The drawing under review shows one solid part. Ordinate dimensions are in mm from its lowest x, y, z. Round coordinates to 2 decimals unless told otherwise and drop trailing zeros. Order: outer loops, then holes, each group sorted by start corner. A loop starts at its lowest first (then second) coordinate and runs counter-clockwise, first axis right, second up. Notation, with made-up numbers: M 76,74 L 108,74 A20 cw 108,105 Z; hole C 74.5,-4 d9. An arc over 180 degrees is marked long. Write item = value, one per line. Start each with the question number.
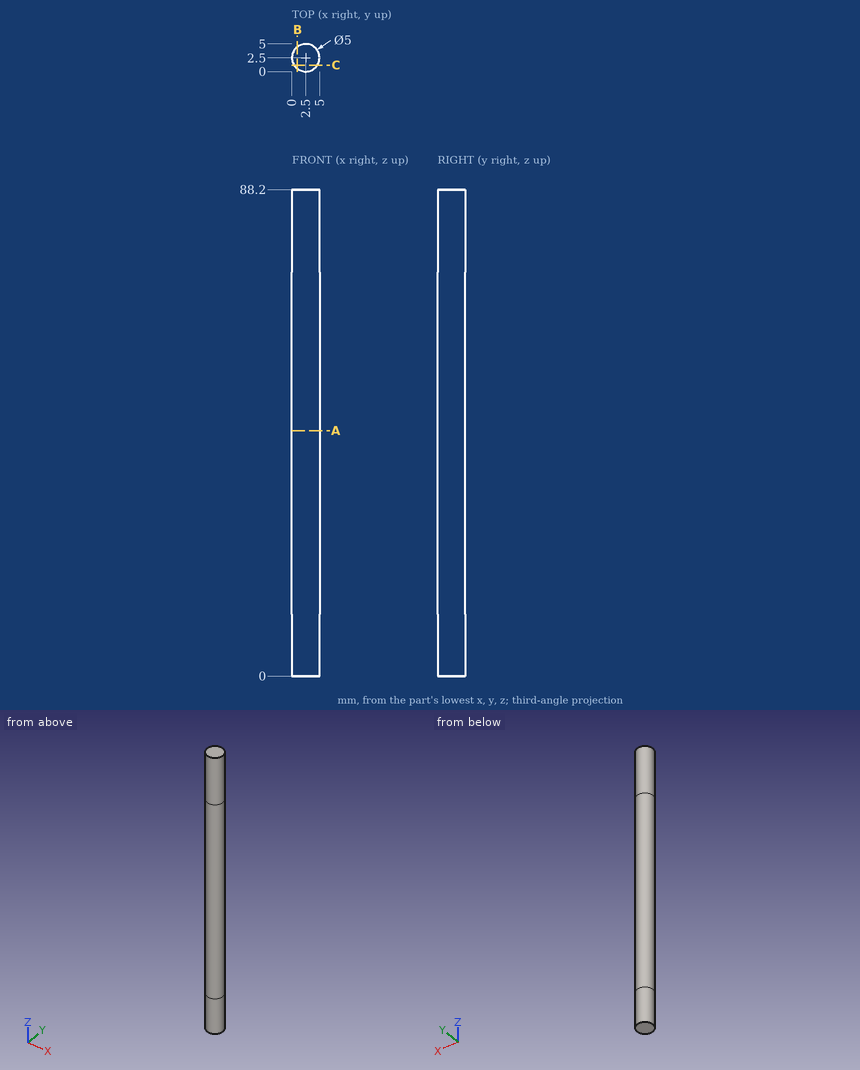
(1) Consider section C-C, the plane y = 1.15. Write out the cut boundary in (x, z), then the cut area to 3 significant figures.
(2) For line 1 along Y through (x, z) = (2.65, 65.5); line 2 along X through (y, z) = (1, 52); line 3 along X through (y, z) = (3.4, 32), list the stretches that pass through material, from the lowest coordinate up. Write a range as [from, to].
(3) Consider section B-B, the plane x = 1. Write out the cut boundary in (y, z), then the cut area to 3 significant figures.
(4) Consider section A-A, the plane z = 44.5. Write out the cut boundary in (x, y), then the cut area to 3 significant figures.
Completed:
q1.outline = M 0.4,0 L 4.6,0 L 4.6,88.2 L 0.4,88.2 Z
q1.area = 371 mm2
q2.line_1 = [0, 5]
q2.line_2 = [0.5, 4.5]
q2.line_3 = [0.17, 4.83]
q3.outline = M 0.5,0 L 4.5,0 L 4.5,88.2 L 0.5,88.2 Z
q3.area = 353 mm2
q4.outline = C 2.5,2.5 d5
q4.area = 19.6 mm2
